CAD build for the part. Positions are in the model's coordinates, mm. A direction names the side the tool comes from. Give positions to 0.01 mm unless a question says otherwise; leave off trailing zeros. Loops run counter-clockwise (first coordinate to the right, second up) from the corner with the lowest first, then second, coordinate; pieces in that order, holes last. Notation, with made-up numbers: M -1,64.25 L 17,64.25 A23 ccw 17,74.25 Z; hole C -34,-26.5 d3. An arc over 180 degrees is marked long. One line per question, with ' | ' between items.
```python
from build123d import *

# Parameters (mm, degrees)
BOSS_EXTRUDE1_DEPTH = 4.7625
SKETCH2_W           = 3.2
SKETCH2_H           = 9.625
SKETCH2_H_2         = 2.75
SKETCH2_W_2         = 1.15
CUT_EXTRUDE1_DEPTH  = 4.7625


with BuildPart() as part:
    # Sketch1 → Boss-Extrude1 (new body)
    with BuildSketch(Plane(origin=(0, 0, 0), x_dir=(1, 0, 0), z_dir=(0, 1, 0))):
        Polygon((-25.4, -63.5), (-25.4, 63.5), (-25.4, 68.2625), (-19.05, 68.2625), (-19.05, 63.5), (-2.4, 63.5), (-2.4, -3), (2.4, -3), (2.4, 63.5), (19.05, 63.5), (19.05, 68.2625), (25.4, 68.2625), (25.4, 63.5), (25.4, -63.5), (25.4, -68.2625), (19.05, -68.2625), (19.05, -63.5), (-19.05, -63.5), (-19.05, -68.2625), (-25.4, -68.2625), align=None)
    extrude(amount=BOSS_EXTRUDE1_DEPTH)

    # Sketch2 → Cut-Extrude1 (cut)
    with BuildSketch(Plane(origin=(0, 4.7625, 0), x_dir=(1, 0, 0), z_dir=(0, 1, 0))):
        with Locations((-10.725, 58.6875)):
            Rectangle(SKETCH2_W, SKETCH2_H)
        with Locations((-10.725, 52.5)):
            Rectangle(SKETCH2_W, SKETCH2_H_2)
        with Locations((-8.55, 52.5)):
            Rectangle(SKETCH2_W_2, SKETCH2_H_2)
        with Locations((-10.725, 46.3125)):
            Rectangle(SKETCH2_W, SKETCH2_H)
        with Locations((-12.9, 52.5)):
            Rectangle(SKETCH2_W_2, SKETCH2_H_2)
        with Locations((10.725, 58.6875)):
            Rectangle(SKETCH2_W, SKETCH2_H)
        with Locations((10.725, 52.5)):
            Rectangle(SKETCH2_W, SKETCH2_H_2)
        with Locations((8.55, 52.5)):
            Rectangle(SKETCH2_W_2, SKETCH2_H_2)
        with Locations((12.9, 52.5)):
            Rectangle(SKETCH2_W_2, SKETCH2_H_2)
        with Locations((10.725, 46.3125)):
            Rectangle(SKETCH2_W, SKETCH2_H)
        with Locations((-10.725, -46.3125)):
            Rectangle(SKETCH2_W, SKETCH2_H)
        with Locations((-10.725, -58.6875)):
            Rectangle(SKETCH2_W, SKETCH2_H)
        with Locations((-12.9, -52.5)):
            Rectangle(SKETCH2_W_2, SKETCH2_H_2)
        with Locations((-10.725, -52.5)):
            Rectangle(SKETCH2_W, SKETCH2_H_2)
        with Locations((-8.55, -52.5)):
            Rectangle(SKETCH2_W_2, SKETCH2_H_2)
        with Locations((10.725, -46.3125)):
            Rectangle(SKETCH2_W, SKETCH2_H)
        with Locations((8.55, -52.5)):
            Rectangle(SKETCH2_W_2, SKETCH2_H_2)
        with Locations((10.725, -52.5)):
            Rectangle(SKETCH2_W, SKETCH2_H_2)
        with Locations((12.9, -52.5)):
            Rectangle(SKETCH2_W_2, SKETCH2_H_2)
        with Locations((10.725, -58.6875)):
            Rectangle(SKETCH2_W, SKETCH2_H)
    extrude(amount=-CUT_EXTRUDE1_DEPTH, mode=Mode.SUBTRACT)


solid = part.part
```
Item 1: Saw through at B-B on z = 43.5. Give the cut face in (x, y) (1 decimal), and give its area (3 significant figures).
Conclusion:
outline: M -25.4,0 L -12.3,0 L -12.3,4.8 L -25.4,4.8 Z; M -9.1,0 L 9.1,0 L 9.1,4.8 L -9.1,4.8 Z; M 12.3,0 L 25.4,0 L 25.4,4.8 L 12.3,4.8 Z | area: 211 mm²
Item 2: 3-axis set-ups, long thin cutter, end or side, ignore diameter. For faces 1 (the flat face through (9.125, 2, 46)), 2 (the flat face through (-13.475, 2, 53)), 3 (the flat face through (11, 2, -41.5)): which of +Z, -Z, +X, -X, +Y, -Y reach the whole face in a straight line?
Conclusion:
face 1: +Z, +Y, -Y | face 2: +Y, -Y | face 3: -Z, +Y, -Y
Item 3: Drop flat-ended pins along their axis: P1, Ø1.3, axis at x = 8.5, y = 1.5, coming from the +Z side; P2, Ø0.9, axis at x = 13, y = 2, coming from the -Z side. Give the stop position or say it passes through.
Conclusion:
P1: z = 63.5 | P2: z = -63.5
Item 4: Drill centre lines: line 1 along Z through (x, y) = (9, 1.7) (3 decimals); line 2 along X through (y, z) = (4.15, -61.5) (3 decimals); line 3 along X through (y, z) = (1.9, 50.5) (3 decimals). Where is each one in solid material? Low to high. Write a range as [from, to].
Conclusion:
line 1: [-63.5, -53.875], [-51.125, 51.125], [53.875, 63.5] | line 2: [-25.4, -12.325], [-9.125, -2.4], [2.4, 9.125], [12.325, 25.4] | line 3: [-25.4, -12.325], [-9.125, 9.125], [12.325, 25.4]
Item 5: Mould opens along X. For faces 4 (the flat face through (-13.475, 2, -52)), 5 (the flat face through (-22, 2, 68.262)) say: pulls with the +X half, pulls with the -X half, needs draft (parallel to the pull), parting line crosses it, or undercut.
Conclusion:
face 4: undercut | face 5: needs draft
Item 6: Saw through at A-A on z = -13. Give the cut face in (x, y), and give its area (3 significant figures).
Conclusion:
outline: M -25.4,0 L -2.4,0 L -2.4,4.76 L -25.4,4.76 Z; M 2.4,0 L 25.4,0 L 25.4,4.76 L 2.4,4.76 Z | area: 219 mm²
Item 7: Saw through at C-C on x = 16. Give the cut face in (y, z), and give its area (3 significant figures).
Conclusion:
outline: M 0,-63.5 L 4.76,-63.5 L 4.76,63.5 L 0,63.5 Z | area: 605 mm²
